Source: CAD feature listing. Evaluate the final solid. Frame: model axes, mm. Face numbers are marked on the shaded views. A direction names the side the tool comes from. Round coordinates to 2 decimals unless told otherwise and drop trailing zeros. Order: outer loops, then holes, each group sorted by start corner. A loop starts at its lowest first (then second) coordinate and runs counter-clockwise, first axis right, second up. Notation, with made-up numbers: (6.25, -38.5) -> (28.25, -38.5) arc R18 ccw to (28.25, -15.5) -> close; hole circle Ø7 at (68, 33.25). An arc over 180 degrees is marked (long way). Answer as CSV lines item,"result". Start each with the question number.
(1) Section query B-B (y = 0). Output: boundary loops of the cut face in (x, z) (3 decimals).
(2) Contact query for flat-ended pins moving along their axis: P1, Ø1.6, axis at y = -13, z = 3, coming from the +X side; P2, Ø1.9, axis at y = -11, z = 2.5, coming from the -X side; P3, Ø1, axis at y = -11.5, z = 4.5, coming from the +X side. Output: stop coordinate, or through.
(3) Section query D-D (z = 1). Count the separate pieces of the cut face and the enclosed holes in it, plus the area to 3 significant figures.
(4) Set-up query: the marked faces 5, 6, 7, 8 and 9. Return all of +Z, -Z, +X, -X, +Y, -Y with unobstructed straight access to the full face (end or side cutting, diameter ignored); none if empty.
(5) Line query: line 1 along Y through (x, z) = (14.5, 2.25) (3 decimals); line 2 along Y through (x, z) = (21.25, 1.5); line 3 along X through (y, z) = (-7, 5). Output: solid intervals per line, ascending. Write a range as from..to.
(6) Section query C-C (x = 0). Output: boundary loops of the cut face in (y, z).
(7) Pull-direction query (X, two-part tool) for the marked faces 1, 2, 3 and 4; classes: +X half, -X half, draft (parallel to the pull), parting line (faces both ways), or undercut.
(8) Section query A-A (x = -21.25). Output: boundary loops of the cut face in (y, z), plus the area to 3 significant figures.
```python
from build123d import *

# Parameters (mm, degrees)
F0_W           = 6.35
F0_H           = 15
F0_W_2         = 16.3
F0_H_2         = 4
F1_DEPTH       = 6.35
F2_D           = 2.05
F3_D           = 2.5
F4_R           = 2.5
F7_D           = 2.05
F7_DEPTH       = 6
F7_TIP         = 0.6158821345
F7_ON_F5_D     = 2.05
F7_ON_F5_DEPTH = 6
F7_ON_F5_TIP   = 0.6158821345
F8_D           = 2


# Not quite as in the source:
# - a length typed as a fraction of an inch, garbled in the dataset ("3 / 203.2 mm" for 3/8 in), is restored
# - a feature names something its author has since deleted; it is built from what else it names


with BuildPart() as f1:
    # F0 (on Top) → F1 (new body)
    with BuildSketch(Plane.XY):
        Polygon((-18.5, 10), (-34.8, 10), (-34.8, 7.5), (-34.8, -7.5), (-34.8, -10), (-18.5, -10), (-14.5, -10), (-11.8, -10), (-10.5, -10), (10.5, -10), (14.5, -10), (18.5, -10), (29.35, -10), (29.35, 10), (18.5, 10), (14.5000000137, 10), (10.5, 10), (-10.5, 10), (-14.5, 10), align=None)
        with Locations((-37.975, 0)):
            Rectangle(F0_W, F0_H)
        with BuildLine():
            Line((-18.5, 14), (-18.5, 10))
            Line((-18.5, 10), (-14.5, 10))
            ThreePointArc((-14.5, 10), (-17.3284271247, 11.1715728753), (-18.5, 14))
        make_face()
        with BuildLine():
            ThreePointArc((-10.5, 14), (-11.6715728753, 11.1715728753), (-14.5, 10))
            Line((-14.5, 10), (-10.5, 10))
            Line((-10.5, 10), (-10.5, 14))
        make_face()
        with BuildLine():
            ThreePointArc((-18.5, 14), (-17.3284271247, 11.1715728753), (-14.5, 10))
            ThreePointArc((-14.5, 10), (-11.6715728753, 11.1715728753), (-10.5, 14))
            Line((-10.5, 14), (-18.5, 14))
        make_face()
        with BuildLine():
            ThreePointArc((-10.5, 14), (-14.5, 18), (-18.5, 14))
            Line((-18.5, 14), (-10.5, 14))
        make_face()
        with BuildLine():
            Line((10.5, 14), (10.5, 10))
            Line((10.5, 10), (14.5000000137, 10))
            ThreePointArc((14.5000000137, 10), (11.6715728801, 11.1715728704), (10.5, 14))
        make_face()
        with BuildLine():
            ThreePointArc((10.5, 14), (11.6715728801, 11.1715728704), (14.5000000137, 10))
            ThreePointArc((14.5000000137, 10), (17.3284271296, 11.1715728801), (18.5, 14))
            ThreePointArc((18.5, 14), (14.5, 18), (10.5, 14))
        make_face()
        with BuildLine():
            ThreePointArc((18.5, 14), (17.3284271296, 11.1715728801), (14.5000000137, 10))
            Line((14.5000000137, 10), (18.5, 10))
            Line((18.5, 10), (18.5, 14))
        make_face()
        with BuildLine():
            ThreePointArc((18.5, -14), (17.3284271247, -11.1715728753), (14.5, -10))
            ThreePointArc((14.5, -10), (11.6715728753, -11.1715728753), (10.5, -14))
            ThreePointArc((10.5, -14), (14.5, -18), (18.5, -14))
        make_face()
        with BuildLine():
            Line((18.5, -14), (18.5, -10))
            Line((18.5, -10), (14.5, -10))
            ThreePointArc((14.5, -10), (17.3284271247, -11.1715728753), (18.5, -14))
        make_face()
        with BuildLine():
            Line((14.5, -10), (10.5, -10))
            Line((10.5, -10), (10.5, -14))
            ThreePointArc((10.5, -14), (11.6715728753, -11.1715728753), (14.5, -10))
        make_face()
        with BuildLine():
            ThreePointArc((-10.5, -14), (-11.6715728753, -11.1715728753), (-14.5, -10))
            ThreePointArc((-14.5, -10), (-17.3284271247, -11.1715728753), (-18.5, -14))
            ThreePointArc((-18.5, -14), (-14.5, -18), (-10.5, -14))
        make_face()
        with BuildLine():
            Line((-11.8, -10), (-14.5, -10))
            ThreePointArc((-14.5, -10), (-11.6715728753, -11.1715728753), (-10.5, -14))
            Line((-10.5, -14), (-10.5, -10))
            Line((-10.5, -10), (-11.8, -10))
        make_face()
        with BuildLine():
            Line((-14.5, -10), (-18.5, -10))
            Line((-18.5, -10), (-18.5, -14))
            ThreePointArc((-18.5, -14), (-17.3284271247, -11.1715728753), (-14.5, -10))
        make_face()
        with Locations((-26.65, 12)):
            Rectangle(F0_W_2, F0_H_2)
        with Locations((-26.65, -12)):
            Rectangle(F0_W_2, F0_H_2)
    extrude(amount=F1_DEPTH)

    # F2 (through all)
    with Locations(Plane(origin=(0, 0, 0), x_dir=(1, 0, 0), z_dir=(0, 0, -1))):
        with Locations((-14.5, -14), (14.5, -14), (14.5, 14), (-14.5, 14)):
            Hole(F2_D / 2)

    # F3 (through all)
    with Locations(Plane(origin=(0, 0, 0), x_dir=(1, 0, 0), z_dir=(0, 0, -1))):
        with Locations((-27.175, 0)):
            Hole(F3_D / 2)

    # F4
    f4_edges = [f1.edges().sort_by_distance(p)[0] for p in [
        (-10.5, 10, 3.175),
        (10.5, 10, 3.175),
        (18.5, 10, 3.175),
        (-10.5, -10, 3.175),
        (10.5, -10, 3.175),
        (18.5, -10, 3.175),
        (-10.5, 14, 3.175),
    ]]
    fillet(f4_edges, radius=F4_R)

    # F7
    with Locations(Plane(origin=(-34.8, 0, 0), x_dir=(0, -1, 0), z_dir=(-1, 0, 0))):
        with Locations((-11.25, 3.175)):
            Hole(F7_D / 2, depth=F7_DEPTH)
            with Locations((0, 0, -(F7_DEPTH + F7_TIP / 2))):  # 118° drill point
                Cone(0, F7_D / 2, F7_TIP, mode=Mode.SUBTRACT)

    # F7 on F5
    with Locations(Plane(origin=(-34.8, 0, 0), x_dir=(0, -1, 0), z_dir=(-1, 0, 0))):
        with Locations((11.25, 3.175)):
            Hole(F7_ON_F5_D / 2, depth=F7_ON_F5_DEPTH)
            with Locations((0, 0, -(F7_ON_F5_DEPTH + F7_ON_F5_TIP / 2))):  # 118° drill point
                Cone(0, F7_ON_F5_D / 2, F7_ON_F5_TIP, mode=Mode.SUBTRACT)

    # F8 (through all)
    with Locations(Plane(origin=(0, 0, 0), x_dir=(1, 0, 0), z_dir=(0, 0, -1))):
        with Locations((-21.25, -7.25), (-21.25, 7.25), (0, 0), (21.25, -7.25), (21.25, 7.25)):
            Hole(F8_D / 2)


solid = f1.part
```
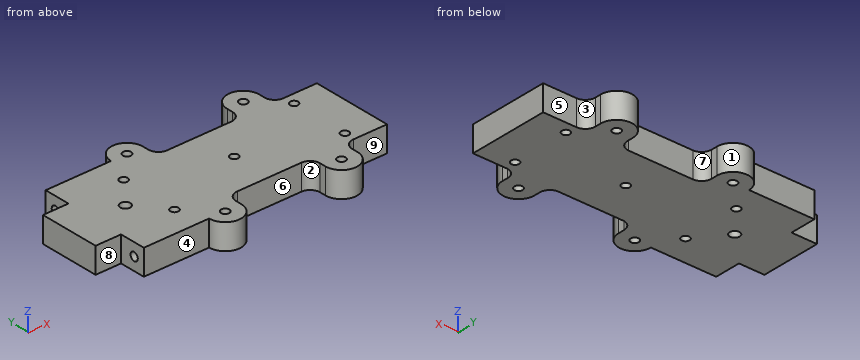
Answer block:
1,outline,"(-41.15, 0) -> (-28.425, 0) -> (-28.425, 6.35) -> (-41.15, 6.35) -> close; (-25.925, 0) -> (-1, 0) -> (-1, 6.35) -> (-25.925, 6.35) -> close; (1, 0) -> (29.35, 0) -> (29.35, 6.35) -> (1, 6.35) -> close"
2,P1,"x = 18.52"
2,P2,"x = -34.8"
2,P3,"x = 19"
3,separate pieces,"1"
3,enclosed holes,"10"
3,area,"1,710 mm2"
4,face 5,"+Z, -Z, +X, +Y"
4,face 6,"+Z, -Z, -Y"
4,face 7,"+Z, -Z, +Y"
4,face 8,"+Z, -Z, -X, -Y"
4,face 9,"+Z, -Z, +X, -Y"
5,line 1,"-18..-15.025, -12.975..12.975, 15.025..18"
5,line 2,"-10..-8.25, -6.25..6.25, 8.25..10"
5,line 3,"-41.15..-22.22, -20.28..20.28, 22.22..29.35"
6,outline,"(-10, 0) -> (-1, 0) -> (-1, 6.35) -> (-10, 6.35) -> close; (1, 0) -> (10, 0) -> (10, 6.35) -> (1, 6.35) -> close"
7,face 1,"undercut"
7,face 2,"undercut"
7,face 3,"+X half"
7,face 4,"draft"
8,outline,"(-14, 0) -> (-8.25, 0) -> (-8.25, 6.35) -> (-14, 6.35) -> close; (-6.25, 0) -> (6.25, 0) -> (6.25, 6.35) -> (-6.25, 6.35) -> close; (8.25, 0) -> (14, 0) -> (14, 6.35) -> (8.25, 6.35) -> close"
8,area,"152 mm2"
